Autodesk Inventor part; units mm, degrees
ref_plane "YZ Plane" through (0, 0, 0) normal (1, 0, 0) x (0, 1, 0)
ref_plane "XZ Plane" through (0, 0, 0) normal (0, 1, 0) x (-1, 0, 0)
ref_plane "XY Plane" through (0, 0, 0) normal (0, 0, 1) x (1, 0, 0)
sketch "Sketch1" plane through (0, 0, 0) normal (0, 0, 1) x (1, 0, 0)
  line L0 (0, 0) -> (25, 0)
  line L1 (25, 0) -> (25, 25)
  line L2 (25, 25) -> (0, 25)
  line L3 (0, 25) -> (0, 0)
  line L4 (3, 22) -> (22, 22)
  line L5 (22, 22) -> (22, 3)
  line L6 (22, 3) -> (3, 3)
  line L7 (3, 3) -> (3, 22)
  dimension "d0" = 25
  dimension "d1" = 25
  dimension "d2" = 3
extrude "Extrusion1" add sketch "Sketch1" against normal blind 300
sketch "Sketch2" plane through (25, 0, 0) normal (1, 0, 0) x (0, 0, -1)
  line L0 (0, 0) -> (0, 25)
  line L1 (0, 0) -> (300, 0)
  line L2 (300, 25) -> (300, 0)
  line L3 (0, 25) -> (300, 25)
  line L4 (0, 25) -> (300, 25)
  line L5 (48.3423, 25) -> (60, 0)
  line L6 (0, 0) -> (300, 0)
  line L7 (0, 0) -> (-11.6577, 25)
  line L8 (-11.6577, 25) -> (48.3423, 25)
  line L9 (255, 0) -> (230, 25)
  line L10 (255, 0) -> (300, 0)
  line L11 (0, 3) -> (300, 3)
  line L12 (275, 25) -> (230, 25)
  line L13 (255, 0) -> (255, 25)
  line L14 (242.5, 12.5) -> (255, 25)
  line L15 (255, 0) -> (255, 3)
  line L16 (0, 3) -> (300, 3)
  line L17 (252, 3) -> (255, 3)
  line L18 (252, 3) -> (255, 0)
  point P0 (58.6011, 3)
  point P1 (255, 3)
  point P2 (255, 3)
  dimension "d6" = 65
  dimension "d10" = 60
  dimension "d11" = 45
  dimension "d21" = 70
extrude "Extrusion2" cut sketch "Sketch2" against normal blind 300 contours L13 L11 L2 L1 | L13 L3 L2 L11 keep common part
properties part number "P601" material "Aluminum 6061"
The listing builds one solid part. Answer for the finished solid, in the listing's coordinates (mm). A direction names the side the tool comes from. Coordinates: 2 decimals unless noted, no trailing zeros. Write each loop counter-clockwise with the first axis right and the second up, starting at its lowest first coordinate (ties: lowest second). Pieces come first, ordered by that corner, then holes. Notation, with made-up numbers: M 27.5,83 L 53.5,83 A37 cw 53.5,120 Z; hole C 72,85.5 d6. An arc over 180 degrees is marked long. Write each question's results on one line, items separated by ' | '.
Item 1: Which of the six approach directions +Z, -Z, +X, -X, +Y, -Y give full straight-line access (tool end or side, diameter ignored) to faces 4 (the face through (25, 12, -277)), 5 (the face through (3, 12, -277))?
Answer below:
face 4: +Z, -Z, +X, +Y, -Y | face 5: +Z, -Z
Item 2: The part is cut by section A-A on x = 16.25. Determine the outline of the cut face in (y, z), and give its area (3 significant figures).
Answer below:
outline: M 0,-300 L 3,-300 L 3,-255 L 0,-255 Z; M 22,-300 L 25,-300 L 25,-255 L 22,-255 Z | area: 270 mm2
Item 3: For a pull along X with two mould halves and no side action, classify faces 1 (the face through (0, 13, -277)), 2 (the face through (13, 23, -255)), 3 (the face through (13, 3, -277)) as released by +X, released by -X, zero draft, split by the parting line, or undercut.
Answer below:
face 1: released by -X | face 2: zero draft | face 3: undercut
Item 4: Consider probe 1 along Y at (x, z) = (3.5, -271). Determine where the line is inside the solid, lowest interval first. Write a range as [from, to].
Answer below:
probe 1: [0, 3], [22, 25]
Item 5: The part is cut by section C-C on z = -284. Determine the outline of the cut face in (x, y).
Answer below:
outline: M 0,0 L 25,0 L 25,25 L 0,25 Z; hole M 3,3 L 22,3 L 22,22 L 3,22 Z
